Drawing for the job (mm, zero at the part's lowest x, y, z). A direction names the side the tool comes from. Coordinates: 2 decimals unless noted, no trailing zeros. Write each loop counter-clockwise with the first axis right and the second up, starting at its lowest first coordinate (ties: lowest second). Pieces come first, ordered by that corner, then holes. Notation, with made-up numbers: M -19,-36 L 17,-36 A12 cw 17,-31 Z; hole C 76,37 d2. An arc over 180 degrees is marked long. Use a Markdown table: item, result. Add a question column.
Q1. Tool access for the marked faces 1, 2, 3 and 4: list every direction of +Z, -Z, +X, -X, +Y, -Y with a clear straight run to the whole face (end or side of a thin tool).
Q2. Wall check: L1, parallel to Z at x = 11, y = 0.55; L2, parallel to Y at x = 11, z = 9.2; L3, parallel to X at y = 0.4, z = 7. Give the ranges that are in metal, low to high. Write a range as from..to.
Q3. Slice it at D-D on z = 1. Write the cut outline in (x, y), then the cut area to 3 significant figures.
Q4. Pin check, flat tips, straight feed: pin 1 Ø1 at (x, y) = (4.5, 4) entering from -Z; pin 2 Ø1.4 at (x, y) = (11, 6) entering from +Z; pin 3 Ø1.8 at (x, y) = (2, 4.5) entering from +Z; pin 4 Ø1.5 at (x, z) = (15, 8.5) entering from -Y. Stop position of each tip, or through.
Q5. Slice it at C-C on x = 3. Write the cut outline in (y, z), then the cut area to 4 significant figures.
Q6. Slice it at B-B on y = 0.75. Write the cut outline in (x, z).
Q7. Mould opens along X. For the marked faces 5, 6, 7 and 8 say: released by +X, released by -X, zero draft, split by the parting line, or undercut.
Q8. Slice it at A-A on y = 4.5. Write the cut outline in (x, z), then the cut area to 3 significant figures.
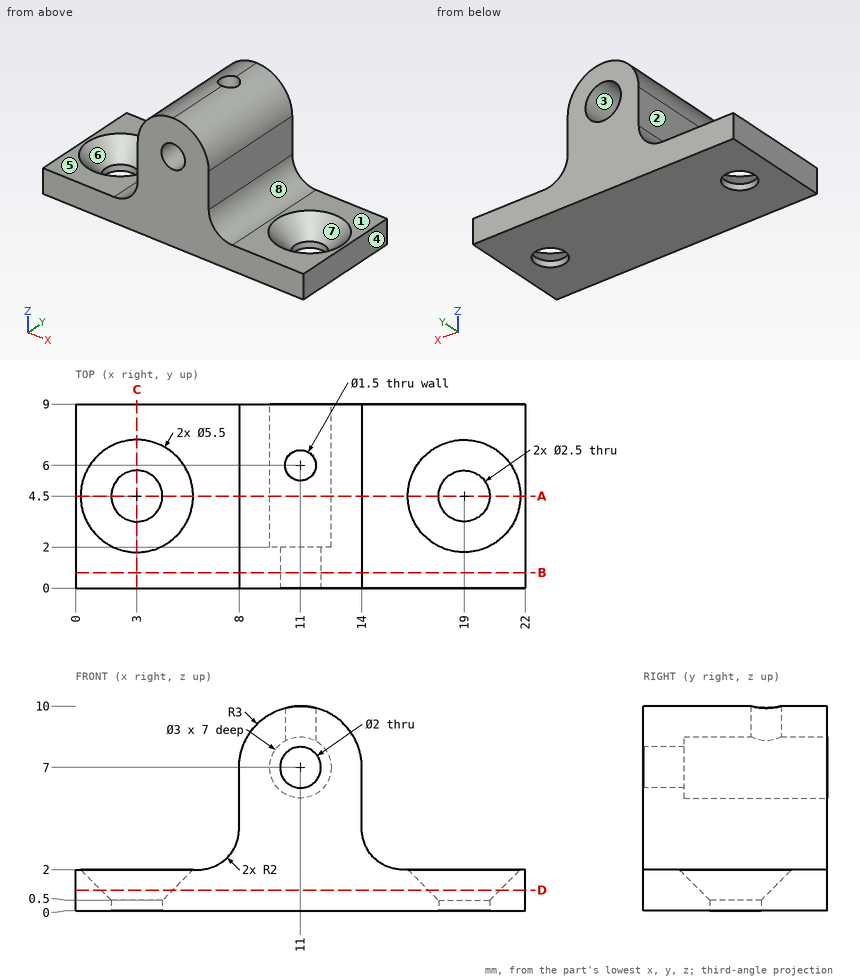
Recorded:
| question | item | result |
|---|---|---|
| 1 | face 1 | +Z, +X, +Y, -Y |
| 1 | face 2 | +Z, -X, +Y, -Y |
| 1 | face 3 | +Y |
| 1 | face 4 | +Z, -Z, +X, +Y, -Y |
| 2 | L1 | 0..6, 8..10 |
| 2 | L2 | 0..5.25, 6.75..9 |
| 2 | L3 | 8..10, 12..14 |
| 3 | outline | M 0,0 L 22,0 L 22,9 L 0,9 Z; hole C 3,4.5 d3.5; hole C 19,4.5 d3.5 |
| 3 | area | 179 mm² |
| 4 | pin 1 | z = 0 |
| 4 | pin 2 | z = 5.67 |
| 4 | pin 3 | z = 1.15 |
| 4 | pin 4 | through |
| 5 | outline | M 0,0 L 3.25,0 L 3.25,0.5 L 1.75,2 L 0,2 Z; M 5.75,0 L 9,0 L 9,2 L 7.25,2 L 5.75,0.5 Z |
| 5 | area | 10.75 mm² |
| 6 | outline | M 0,0 L 22,0 L 22,2 L 16,2 A2 cw 14,4 L 14,7 A3 ccw 8,7 L 8,4 A2 cw 6,2 L 0,2 Z; hole C 11,7 d2 |
| 7 | face 5 | zero draft |
| 7 | face 6 | undercut |
| 7 | face 7 | undercut |
| 7 | face 8 | released by +X |
| 8 | outline | M 0,0 L 1.75,0 L 1.75,0.5 L 0.25,2 L 0,2 Z; M 4.25,0 L 17.75,0 L 17.75,0.5 L 16.25,2 L 16,2 A2 cw 14,4 L 14,7 A3 ccw 8,7 L 8,4 A2 cw 6,2 L 5.75,2 L 4.25,0.5 Z; M 20.25,0 L 22,0 L 22,2 L 21.75,2 L 20.25,0.5 Z; hole C 11,7 d3 |
| 8 | area | 68.3 mm² |
